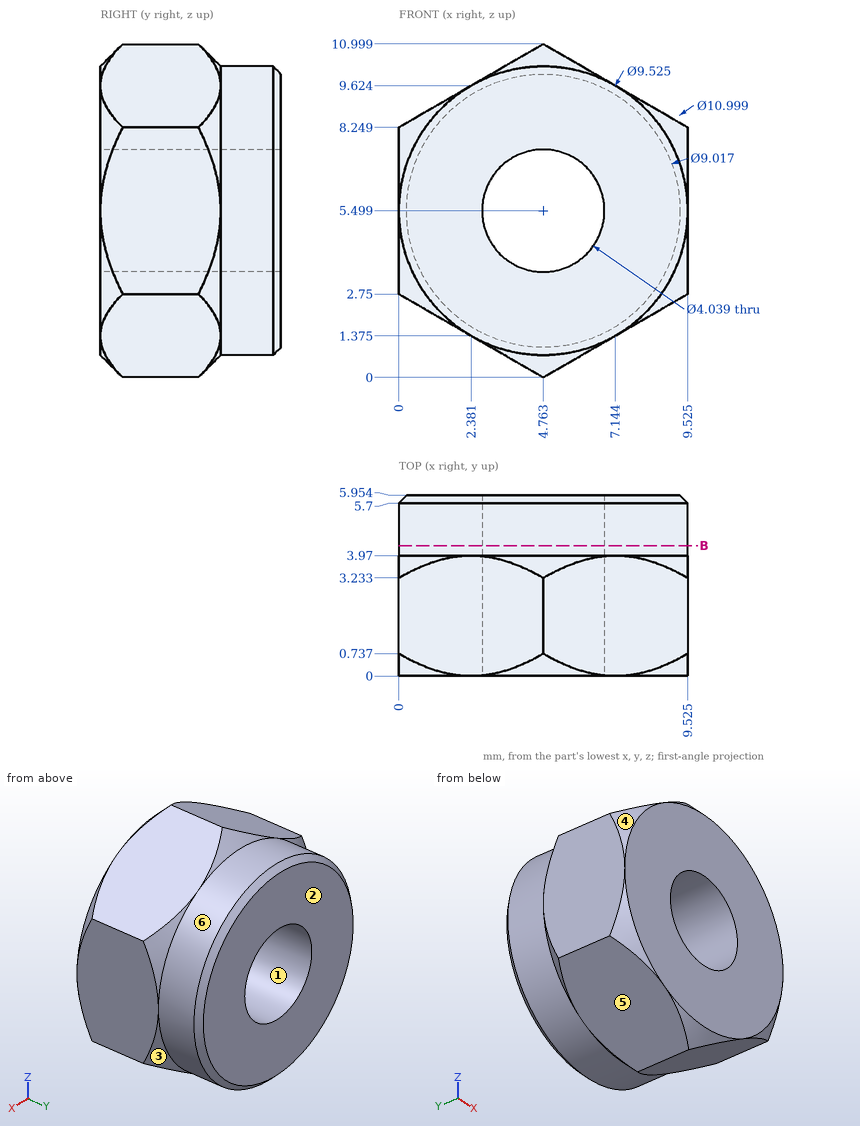
Study the drawing (mm; zero at the part's minimum x, y, z) and answer. A direction names the side the tool comes from. Give positions to 0.01 mm unless a question says otherwise; leave off trailing zeros. Order: outer loops, then holes, each group sorted by start corner. A loop starts at its lowest first (then second) coordinate and runs counter-clockwise, first axis right, second up. Notation, with made-up numbers: (20, 40.25) - (61, 40.25) arc R33 cw to (61, 71.25) - close; hole circle Ø11 at (36, 35). An arc over 180 degrees is marked (long way). Answer as CSV lines item,"result". Start each with the question number.
Q1. The part is cut by section B-B (y = 4.3). Write down the section's boundary in (x, z) (1 decimal).
Q2. Find the intervals of material crossed by L1, parallel to Z at x = 5.5, y = 4.45 (1 decimal); L2, parallel to X at y = 1.95, z = 6 (1 decimal); L3, parallel to Z at x = 5.5, y = 1.45 (1 decimal), in increasing order. Write a range as [from, to].
Q3. For the marked faces 5 and 6, determine the directions among +Z, -Z, +X, -X, +Y, -Y from which every point of the face is accessible in a straight line to the end or side of a thin tool.
Q4. Given pin 1 Ø2 at (x, y) = (7.5, 2.5) entering from -Z; pin 2 Ø2 at (x, y) = (1.5, 3) entering from +Z; pin 3 Ø1.5 at (y, z) = (4, 1.5) entering from -X (1 decimal), each flat-ended and moving along its own axis, determine where each tip first touches the part or whether it passes through.
Q5. The mould has two halves that part along Z. Classify the marked faces 1, 2, 3 and 4: +Z half, -Z half, draft (parallel to the pull), parting line (faces both ways), or undercut.
Check result:
1,outline,"circle Ø9.5 at (4.8, 5.5); hole circle Ø4 at (4.8, 5.5)"
2,L1,"z = [0.8, 3.6], [7.4, 10.2]"
2,L2,"x = [0, 2.8], [6.7, 9.5]"
2,L3,"z = [0.4, 3.6], [7.4, 10.6]"
3,face 5,"-Z, -X, +Y, -Y"
3,face 6,"+Y"
4,pin 1,"stops at z = 1"
4,pin 2,"stops at z = 9.69"
4,pin 3,"stops at x = 1"
5,face 1,"undercut"
5,face 2,"draft"
5,face 3,"-Z half"
5,face 4,"+Z half"
